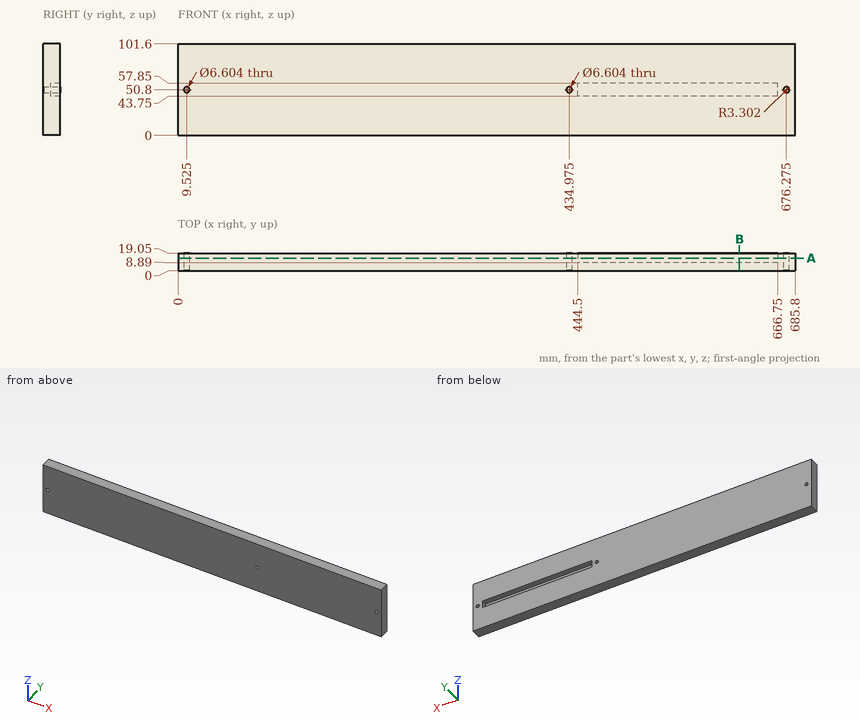
Check sheet for the drawn part. Datum: minimum x, y, z corner. Units: mm. Give positions to 0.01 mm unless a question says otherwise; leave off trailing zeros. Order: outer loops, then holes, each group sorted by start corner. A loop starts at its lowest first (then second) coordinate and runs counter-clockwise, first axis right, second up. Notation, with made-up numbers: (17, 51.25) - (39, 51.25) arc R5 ccw to (39, 57.25) - close; hole circle Ø9 at (25.5, -30.5). An arc over 180 degrees is marked (long way). Answer in a Markdown table with one row per item. Add a question column.
Q1. Cross-section at A-A, the plane y = 13.75. Enter the section's corners in (x, z) (3 decimals).
Q2. Cross-section at B-B, the plane x = 624. Enter the section's corners in (y, z), then the cut area to 3 significant figures.
Q3. Material ranges on probe 1 along Z at (x, y) = (562, 16.5); probe 2 along X at (y, z) = (18, 45.5), recorded low to high. Write a range as from..to.
Check values:
| question | item | result |
|---|---|---|
| 1 | outline | (0, 0) - (685.8, 0) - (685.8, 101.6) - (0, 101.6) - close; hole circle Ø6.604 at (9.525, 50.8); hole circle Ø6.604 at (434.975, 50.8); hole (444.5, 43.75) - (666.75, 43.75) - (666.75, 57.85) - (444.5, 57.85) - close; hole (676.275, 47.498) arc R3.302 ccw to (679.577, 50.8) arc R3.302 ccw to (676.275, 54.102) arc R3.302 ccw to start |
| 2 | outline | (0, 0) - (19.05, 0) - (19.05, 43.75) - (8.89, 43.75) - (8.89, 57.85) - (19.05, 57.85) - (19.05, 101.6) - (0, 101.6) - close |
| 2 | area | 1,790 mm^2 |
| 3 | probe 1 | z = 0..43.75, 57.85..101.6 |
| 3 | probe 2 | x = 0..444.5, 666.75..685.8 |
